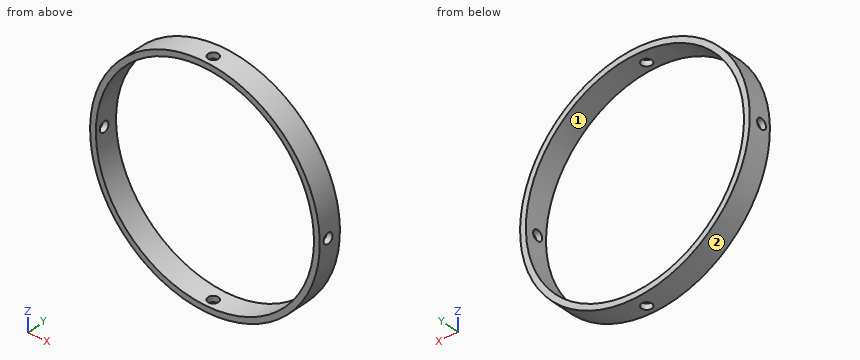
from build123d import *

# Parameters (mm, degrees)
SKETCH1_R           = 37.846
SKETCH1_R_2         = 35.941
BOSS_EXTRUDE1_DEPTH = 7.62
SKETCH2_R           = 1.692869147
CUT_EXTRUDE1_DEPTH  = 86.62
CIRPATTERN1_COUNT   = 4


with BuildPart() as part:
    # Sketch1 → Boss-Extrude1 (new body)
    with BuildSketch(Plane(origin=(0, 0, 0), x_dir=(1, 0, 0), z_dir=(0, 1, 0))):
        with Locations(Location((0, 0, 0), (0, 0, 90))):
            Circle(SKETCH1_R)
        with Locations(Location((0, 0, 0), (0, 0, 90))):
            Circle(SKETCH1_R_2, mode=Mode.SUBTRACT)
    extrude(amount=BOSS_EXTRUDE1_DEPTH)

    # Sketch2 → Cut-Extrude1 (cut)
    with BuildSketch(Plane.XY):
        with Locations(Location((0, 3.171011831, 0), (0, 0, 180))):
            Circle(SKETCH2_R)
    cut_extrude1 = extrude(amount=CUT_EXTRUDE1_DEPTH, mode=Mode.SUBTRACT)

    # CirPattern1: Cut-Extrude1 ×4 about axis
    cirpattern1_axis = Axis((0, 7.62, 0), (0, -1, 0))
    for i in range(1, CIRPATTERN1_COUNT):
        add(cut_extrude1.rotate(cirpattern1_axis, i * 360 / CIRPATTERN1_COUNT), mode=Mode.SUBTRACT)


solid = part.part
Read the model definition and answer for the solid it produces. Units are mm, in the model's axes. Face numbers are marked on the shaded views. Coordinates: 2 decimals unless noted, no trailing zeros. Loops run counter-clockwise (first coordinate to the right, second up) from the corner with the lowest first, then second, coordinate; pieces in that order, holes last. Notation, with made-up numbers: (87.25, 16) -> (109.25, 16) arc R23 ccw to (109.25, 40) -> close; hole circle Ø10 at (-27.5, 45.5). An arc over 180 degrees is marked (long way). Write item = value, one per line. Start each with the question number.
1) The part is cut by section D-D, the plane z = 25.5. Determine the outline of the cut face in (x, y), plus the area to 3 significant figures.
2) The mould has two halves that part along X. Classify the marked faces 1 and 2: pulls with the +X half, pulls with the -X half, needs draft (parallel to the pull), parting line crosses it, or undercut.
3) The part is cut by section A-A, the plane z = 0. Determine the outline of the cut face in (x, y), plus the area to 3 significant figures.
4) Find the intervals of material crossed by L1, parallel to Y at x = -37.1, z = 0; L2, parallel to Z at x = -32, y = 6.75; L3, parallel to Z at x = -19, y = 3.25, in increasing order. Write a range as from..to.
5) Given P1, Ø4.5, axis at x = 0, y = 3.17, coming from the +Z side; P2, Ø1, axis at x = 3, y = 2.5, coming from the -Z side; P3, Ø12, axis at x = -19.5, z = 19.5, coming from the +Y side; P4, Ø1, axis at y = 5.5, z = -23.5, coming from the -X side, each flat-ended and moving along its own axis, determine where each tip first touches the part or whether it passes through.
6) The part is cut by section C-C, the plane x = -24. Determine the outline of the cut face in (y, z).
7) The part is cut by section B-B, the plane x = 0. Determine the outline of the cut face in (y, z), plus the area to 3 significant figures.
Result:
q1.outline = (-27.97, 0) -> (-25.33, 0) -> (-25.33, 7.62) -> (-27.97, 7.62) -> close; (25.33, 0) -> (27.97, 0) -> (27.97, 7.62) -> (25.33, 7.62) -> close
q1.area = 40.2 mm²
q2.face_1 = undercut
q2.face_2 = parting line crosses it
q3.outline = (-37.85, 0) -> (-35.94, 0) -> (-35.94, 1.48) -> (-37.85, 1.48) -> close; (-37.85, 4.86) -> (-35.94, 4.86) -> (-35.94, 7.62) -> (-37.85, 7.62) -> close; (35.94, 0) -> (37.85, 0) -> (37.85, 1.48) -> (35.94, 1.48) -> close; (35.94, 4.86) -> (37.85, 4.86) -> (37.85, 7.62) -> (35.94, 7.62) -> close
q3.area = 16.1 mm²
q4.L1 = 0..1.48, 4.86..7.62
q4.L2 = -20.21..-16.36, 16.36..20.21
q4.L3 = -32.73..-30.51, 30.51..32.73
q5.P1 = 37.85
q5.P2 = -37.76
q5.P3 = through
q5.P4 = -30.06
q6.outline = (0, -29.26) -> (7.62, -29.26) -> (7.62, -26.75) -> (0, -26.75) -> close; (0, 26.75) -> (7.62, 26.75) -> (7.62, 29.26) -> (0, 29.26) -> close
q7.outline = (0, -37.85) -> (1.48, -37.85) -> (1.48, -35.94) -> (0, -35.94) -> close; (0, 35.94) -> (1.48, 35.94) -> (1.48, 37.85) -> (0, 37.85) -> close; (4.86, -37.85) -> (7.62, -37.85) -> (7.62, -35.94) -> (4.86, -35.94) -> close; (4.86, 35.94) -> (7.62, 35.94) -> (7.62, 37.85) -> (4.86, 37.85) -> close
q7.area = 16.1 mm²
